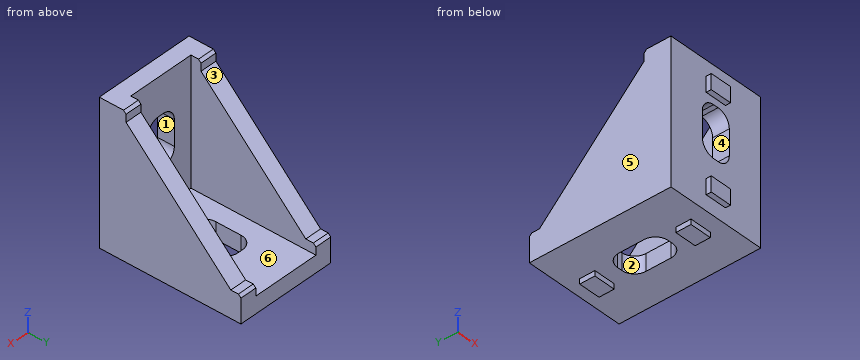
```python
from build123d import *

# Parameters (mm, degrees)
SKETCH1_W           = 20
SKETCH1_H           = 28
BOSS_EXTRUDE1_DEPTH = 3.3
SKETCH2_W           = 20
SKETCH2_H           = 24.7
BOSS_EXTRUDE2_DEPTH = 3.3
BOSS_EXTRUDE3_DEPTH = 3.3
BOSS_EXTRUDE4_DEPTH = 3.3
CHAMFER1_SIZE       = 0.5
SKETCH5_W           = 4.3
SKETCH5_H           = 3
BOSS_EXTRUDE5_DEPTH = 1
SKETCH6_W           = 4.3
SKETCH6_H           = 3
BOSS_EXTRUDE6_DEPTH = 1


with BuildPart() as part:
    # Sketch1 → Boss-Extrude1 (new body)
    with BuildSketch(Plane.XY):
        with Locations((10, 14)):
            Rectangle(SKETCH1_W, SKETCH1_H)
        with BuildLine():
            Line((10.5, 9), (9.5, 9))
            ThreePointArc((9.5, 9), (7.732233047, 9.732233047), (7, 11.5))
            Line((7, 11.5), (7, 16.5))
            ThreePointArc((7, 16.5), (7.732233047, 18.267766953), (9.5, 19))
            Line((9.5, 19), (10.5, 19))
            ThreePointArc((10.5, 19), (12.267766953, 18.267766953), (13, 16.5))
            Line((13, 16.5), (13, 11.5))
            ThreePointArc((13, 11.5), (12.267766953, 9.732233047), (10.5, 9))
        make_face(mode=Mode.SUBTRACT)
    extrude(amount=-BOSS_EXTRUDE1_DEPTH)

    # Sketch2 → Boss-Extrude2 (add)
    with BuildSketch(Plane(origin=(0, 0, 0), x_dir=(1, 0, 0), z_dir=(0, 1, 0))):
        with Locations((10, -12.35)):
            Rectangle(SKETCH2_W, SKETCH2_H)
        with BuildLine():
            Line((10.5, -17.35), (9.5, -17.35))
            ThreePointArc((9.5, -17.35), (7.732233047, -16.617766953), (7, -14.85))
            Line((7, -14.85), (7, -9.85))
            ThreePointArc((7, -9.85), (7.732233047, -8.082233047), (9.5, -7.35))
            Line((9.5, -7.35), (10.5, -7.35))
            ThreePointArc((10.5, -7.35), (12.267766953, -8.082233047), (13, -9.85))
            Line((13, -9.85), (13, -14.85))
            ThreePointArc((13, -14.85), (12.267766953, -16.617766953), (10.5, -17.35))
        make_face(mode=Mode.SUBTRACT)
    extrude(amount=BOSS_EXTRUDE2_DEPTH)

    # Sketch3 → Boss-Extrude3 (add)
    with BuildSketch(Plane(origin=(0, 0, 0), x_dir=(0, 0, -1), z_dir=(1, 0, 0))):
        Polygon((0, 28), (-2, 28), (-2, 26), (-22.7, 5.3), (-24.7, 5.3), (-24.7, 3.3), (0, 3.3), align=None)
    extrude(amount=BOSS_EXTRUDE3_DEPTH)

    # Sketch4 → Boss-Extrude4 (add)
    with BuildSketch(Plane(origin=(20, 0, 0), x_dir=(0, 0, -1), z_dir=(1, 0, 0))):
        Polygon((0, 28), (-2, 28), (-2, 26), (-22.7, 5.3), (-24.7, 5.3), (-24.7, 3.3), (0, 3.3), align=None)
    extrude(amount=-BOSS_EXTRUDE4_DEPTH)

    # Chamfer1
    chamfer1_edges = [part.edges().sort_by_distance(p)[0] for p in [
        (1.65, 28, 2),
        (1.65, 5.3, 24.7),
        (18.35, 5.3, 24.7),
        (18.35, 28, 2),
    ]]
    chamfer(chamfer1_edges, length=CHAMFER1_SIZE)

    # Sketch5 → Boss-Extrude5 (add)
    with BuildSketch(Plane(origin=(0, 0, -3.3), x_dir=(-1, 0, 0), z_dir=(0, 0, -1))):
        with Locations((-10, 23.5)):
            Rectangle(SKETCH5_W, SKETCH5_H)
        with Locations((-10, 4.5)):
            Rectangle(SKETCH5_W, SKETCH5_H)
    extrude(amount=BOSS_EXTRUDE5_DEPTH)

    # Sketch6 → Boss-Extrude6 (add)
    with BuildSketch(Plane.XZ):
        with Locations((10, 1.2)):
            Rectangle(SKETCH6_W, SKETCH6_H)
        with Locations((10, 20.2)):
            Rectangle(SKETCH6_W, SKETCH6_H)
    extrude(amount=BOSS_EXTRUDE6_DEPTH)


solid = part.part
```
Check sheet for the modelled part. Datum: model origin and axes. Units: mm. Face numbers are marked on the shaded views. A direction names the side the tool comes from. Give positions to 0.01 mm unless a question says otherwise; leave off trailing zeros. Order: outer loops, then holes, each group sorted by start corner. A loop starts at its lowest first (then second) coordinate and runs counter-clockwise, first axis right, second up. Notation, with made-up numbers: (-25.5, 46) -> (1.5, 46) arc R23 cw to (1.5, 61) -> close; hole circle Ø7 at (-26, -37.5). An arc over 180 degrees is marked (long way). Use CSV: the item, a comma, the result in double quotes. Start each with the question number.
1) Sectioned sample at C-C, the plane x = 17.5. Record the boundary of the cut face in (y, z).
2) Sectioned sample at B-B, the plane z = 5.5. Record the boundary of the cut face in (x, y), plus the area to 3 significant figures.
3) Set-up check for the marked faces 4, 5 and 6: record each of +Z, -Z, +X, -X, +Y, -Y from which the full face is reachable in a straight line by a thin tool's end or side.
4) Mould release check, pull along Z, two halves, no side actions. Record for the marked faces 1, 2 and 3: released by +Z, released by -Z, zero draft, split by the parting line, or undercut.
5) Material ranges on line 1 (X direction, y = 11, z = 8); line 2 (Z direction, x = 2.25, y = 4.75); line 3 (Y direction, x = 5.25, z = -2.25), recorded low to high. Write a range as from..to.
6) Go/stop test with flat-tipped pins: P1, Ø1, axis at x = 5.5, y = 13, coming from the +Z side; P2, Ø0.5, axis at x = 10, y = -0.5, coming from the -Z side; P3, Ø0.8, axis at x = 2, y = 26.5, coming from the +Z side; P4, Ø2, axis at x = 10, z = 16, coming from the +Y side. Record where each tip stops, or that it passes through.
7) Sectioned sample at D-D, the plane z = 16.25. Record the boundary of the cut face in (x, y).
8) Sectioned sample at A-A, the plane y = 14. Record the boundary of the cut face in (x, z), plus the area to 3 significant figures.
Recorded:
1,outline,"(0, -3.3) -> (28, -3.3) -> (28, 1.5) -> (27.5, 2) -> (26, 2) -> (5.3, 22.7) -> (5.3, 24.2) -> (4.8, 24.7) -> (0, 24.7) -> close"
2,outline,"(0, 0) -> (20, 0) -> (20, 22.5) -> (16.7, 22.5) -> (16.7, 3.3) -> (3.3, 3.3) -> (3.3, 22.5) -> (0, 22.5) -> close"
2,area,"193 mm2"
3,face 4,"+Y, -Y"
3,face 5,"+Z, -Z, -X, +Y, -Y"
3,face 6,"+Z, +Y"
4,face 1,"undercut"
4,face 2,"zero draft"
4,face 3,"released by +Z"
5,line 1,"0..3.3, 16.7..20"
5,line 2,"-3.3..24.7"
5,line 3,"0..28"
6,P1,"z = 0"
6,P2,"z = -0.3"
6,P3,"z = 2"
6,P4,"through"
7,outline,"(0, 0) -> (7.43, 0) -> (7.43, 3.3) -> (3.3, 3.3) -> (3.3, 11.75) -> (0, 11.75) -> close; (12.57, 0) -> (20, 0) -> (20, 11.75) -> (16.7, 11.75) -> (16.7, 3.3) -> (12.57, 3.3) -> close"
8,outline,"(0, -3.3) -> (7, -3.3) -> (7, 0) -> (3.3, 0) -> (3.3, 14) -> (0, 14) -> close; (13, -3.3) -> (20, -3.3) -> (20, 14) -> (16.7, 14) -> (16.7, 0) -> (13, 0) -> close"
8,area,"139 mm2"
